Autodesk Inventor part; units mm, degrees
ref_plane "YZ Plane" through (0, 0, 0) normal (1, 0, 0) x (0, 1, 0)
ref_plane "XZ Plane" through (0, 0, 0) normal (0, 1, 0) x (-1, 0, 0)
ref_plane "XY Plane" through (0, 0, 0) normal (0, 0, 1) x (1, 0, 0)
sketch "Sketch1" plane through (0, 0, 0) normal (0, 0, 1) x (1, 0, 0)
  circle A0 centre (-12.7, -31.75) radius 2.1844
  circle A1 centre (127, -31.75) radius 2.1844
  circle A2 centre (-12.7, -95.25) radius 2.1844
  circle A3 centre (127, -95.25) radius 2.1844
  arc A4 (-17.4625, -95.25) -> (-12.7, -100.0125) centre (-12.7, -95.25) ccw
  arc A5 (-9.3324, -28.3824) -> (-17.4625, -31.75) centre (-12.7, -31.75) ccw
  arc A6 (131.7625, -31.75) -> (123.6324, -28.3824) centre (127, -31.75) ccw
  arc A7 (127, -100.0125) -> (131.7625, -95.25) centre (127, -95.25) ccw
  line L0 (-17.4625, -31.75) -> (-17.4625, -95.25)
  line L1 (-12.7, -100.0125) -> (127, -100.0125)
  line L2 (131.7625, -95.25) -> (131.7625, -31.75)
  line L3 (39.3023, -90.4875) -> (-7.9375, -43.2477)
  line L4 (-7.9375, -43.2477) -> (-7.9375, -90.4875)
  line L5 (122.2375, -43.2477) -> (122.2375, -90.4875)
  line L6 (122.2375, -43.2477) -> (74.9977, -90.4875)
  line L7 (57.15, -100.0125) -> (57.15, -90.4875) construction
  line L8 (-7.9375, -90.4875) -> (39.3023, -90.4875)
  line L9 (52.7727, -90.4875) -> (61.5273, -90.4875)
  line L10 (74.9977, -90.4875) -> (122.2375, -90.4875)
  line L11 (86.9273, -65.0875) -> (27.3727, -65.0875)
  line L12 (96.4523, -55.5625) -> (17.8477, -55.5625)
  line L13 (61.5273, -90.4875) -> (86.9273, -65.0875)
  line L14 (96.4523, -55.5625) -> (123.6324, -28.3824)
  line L15 (-9.3324, -28.3824) -> (17.8477, -55.5625)
  line L16 (27.3727, -65.0875) -> (52.7727, -90.4875)
  circle A8 centre (-12.7, -57.15) radius 2.1844
  circle A9 centre (127, -57.15) radius 2.1844
  point P0 (0, 0)
  dimension "d0" = 9.525
  dimension "d8" = 9.525
  dimension "d9" = 25.4
  dimension "d10" = 45
extrude "Extrusion1" add sketch "Sketch1" along normal blind 5.08
fillet "Fillet2" radius 2.54 6 edges at (39.3023, -90.4875, 2.54) (74.9977, -90.4875, 2.54) (122.2375, -43.2477, 2.54) (122.2375, -90.4875, 2.54) (-7.9375, -43.2477, 2.54) (-7.9375, -90.4875, 2.54)
fillet "Fillet3" radius 2.54 6 edges at (27.3727, -65.0875, 2.54) (86.9273, -65.0875, 2.54) (96.4523, -55.5625, 2.54) (17.8477, -55.5625, 2.54) (61.5273, -90.4875, 2.54) (52.7727, -90.4875, 2.54)
properties part number "hoodbrace"
Could you check a few things on this model? Use its own coordinates, in mm. A direction names the side the tool comes from. Coordinates: 2 decimals unless noted, no trailing zeros. Write each loop counter-clockwise with the first axis right and the second up, starting at its lowest first coordinate (ties: lowest second). Pieces come first, ordered by that corner, then holes. Notation, with made-up numbers: (83, 66) - (94, 66) arc R12 ccw to (94, 83) - close; hole circle Ø7 at (32, 53.5). An arc over 180 degrees is marked (long way). Put each result on its own line as item: value. Start each with the question number.
Q1. Which directions (+Z, -Z, +X, -X, +Y, -Y) give clear straight access to the entire face, cutting with the end or side of a thin tool? Please do faces 1 (the flat face through (58, -55.562, 3)), 2 (the flat face through (56, -100.012, 3)), 3 (the cylindrical face through (31.174, -66.617, 2.576)).
Q2. I want a section at B-B on y = -57.15. Write out the boundary of the cut face in (x, z).
Q3. Please list where these lines run through material, in increasing order: L1, parallel to Y at x = -12.7, z = 2.6; L2, parallel to X at y = -51, z = 0.9; L3, parallel to Y at x = 56.5, z = 2.8.
Q4. I want a section at C-C on z = 2.2. Count the separate pieces of the cut face and the enclosed holes in it, plus the area to 3 significant figures.
Q5. Thinking about a two-plate mould opening in Y: for faces 4 (the flat face through (-17.462, -63, 3)), 5 (the cylindrical face through (78.767, -88.881, 2.576)), 6 (the cylindrical face through (-16.03, -98.654, 2.504)), which applies, pulls with the +Y half, pulls with the -Y half, needs draft (parallel to the pull), parting line crosses it, or undercut?
Q6. I want a section at A-A on x = 93. Write out the boundary of the cut face in (y, z).
Q7. I'm going to push a flat-ended pin straight in: P1, Ø1.5, axis at x = 45.5, z = 2.5, coming from the +Y side. Where does the tip first touch, or does it pass through?
Checks:
1. face 1: +Z, -Z, +Y
1. face 2: +Z, -Z, +X, -X, -Y
1. face 3: +Z, -Z
2. outline: (-17.46, 0) - (-14.88, 0) - (-14.88, 5.08) - (-17.46, 5.08) - close; (-10.52, 0) - (-7.94, 0) - (-7.94, 5.08) - (-10.52, 5.08) - close; (5.96, 0) - (108.34, 0) - (108.34, 5.08) - (5.96, 5.08) - close; (122.24, 0) - (124.82, 0) - (124.82, 5.08) - (122.24, 5.08) - close; (129.18, 0) - (131.76, 0) - (131.76, 5.08) - (129.18, 5.08) - close
3. L1: -100.01 to -97.43, -93.07 to -59.33, -54.97 to -33.93, -29.57 to -26.99
3. L2: -17.46 to -7.94, -0.19 to 13.29, 101.01 to 114.49, 122.24 to 131.76
3. L3: -100.01 to -90.49, -65.09 to -55.56
4. separate pieces: 1
4. enclosed holes: 9
4. area: 4,680 mm²
5. face 4: needs draft
5. face 5: undercut
5. face 6: pulls with the -Y half
6. outline: (-100.01, 0) - (-90.49, 0) - (-90.49, 5.08) - (-100.01, 5.08) - close; (-72.49, 0) - (-55.56, 0) - (-55.56, 5.08) - (-72.49, 5.08) - close
7. P1: y = -55.56
